```python
from build123d import *

# Parameters (mm, degrees)
SKETCH1_W           = 175
SKETCH1_H           = 2
BOSS_EXTRUDE1_DEPTH = 40
SKETCH2_W           = 2
SKETCH2_H           = 40
BOSS_EXTRUDE2_DEPTH = 50
SKETCH3_W           = 100
SKETCH3_H           = 25
BOSS_EXTRUDE3_DEPTH = 2
SKETCH4_R           = 2.5
CUT_EXTRUDE1_DEPTH  = 2
SKETCH5_W           = 12
SKETCH5_H           = 12
CUT_EXTRUDE2_DEPTH  = 2
FILLET1_R           = 5
SKETCH6_R           = 1.6
CUT_EXTRUDE3_DEPTH  = 2
BOSS_EXTRUDE4_DEPTH = 48
SHELL1_DEPTH        = 5.751288694
SHELL1_START        = 4
SHELL1_2_DEPTH      = 1.751288694
SHELL1_START_2      = 129
SHELL1_3_DEPTH      = 44
SKETCH8_R           = 5
SKETCH8_R_2         = 2.383029524
CUT_EXTRUDE4_DEPTH  = 44
SKETCH10_W          = 44
SKETCH10_H          = 28
CUT_EXTRUDE5_DEPTH  = 2
BOSS_EXTRUDE5_REACH = 146.017
SKETCH12_W          = 5.470592624
SKETCH12_H          = 9.51694338
SKETCH12_W_2        = 4.594349632
SKETCH12_H_2        = 8.868192378
CUT_EXTRUDE6_DEPTH  = 188.459328922
SKETCH13_W          = 40
SKETCH13_H          = 2
BOSS_EXTRUDE6_DEPTH = 2
SKETCH14_W          = 3
SKETCH14_H          = 2
BOSS_EXTRUDE7_DEPTH = 2
FILLET3_R           = 5
FILLET4_R           = 5


with BuildPart() as part:
    # Sketch1 → Boss-Extrude1 (new body)
    with BuildSketch(Plane.XY):
        with Locations((87.5, 1)):
            Rectangle(SKETCH1_W, SKETCH1_H)
    extrude(amount=BOSS_EXTRUDE1_DEPTH)

    # Sketch2 → Boss-Extrude2 (add)
    with BuildSketch(Plane.XZ):
        with Locations((1, 20)):
            Rectangle(SKETCH2_W, SKETCH2_H)
    extrude(amount=BOSS_EXTRUDE2_DEPTH)

    # Sketch3 → Boss-Extrude3 (add)
    with BuildSketch(Plane.XY.offset(40)):
        with Locations((52, -12.5)):
            Rectangle(SKETCH3_W, SKETCH3_H)
    extrude(amount=-BOSS_EXTRUDE3_DEPTH)

    # Sketch4 → Cut-Extrude1 (cut)
    with BuildSketch(Plane.ZY):
        with Locations((7.5, -8.5)):
            Circle(SKETCH4_R)
        with Locations((32.5, -42.5)):
            Circle(SKETCH4_R)
    extrude(amount=-CUT_EXTRUDE1_DEPTH, mode=Mode.SUBTRACT)

    # Sketch5 → Cut-Extrude2 (cut)
    with BuildSketch(Plane.XY.offset(40)):
        with Locations((21, -12.5)):
            Rectangle(SKETCH5_W, SKETCH5_H)
        with Locations((41, -12.5)):
            Rectangle(SKETCH5_W, SKETCH5_H)
        with Locations((61, -12.5)):
            Rectangle(SKETCH5_W, SKETCH5_H)
        with Locations((81, -12.5)):
            Rectangle(SKETCH5_W, SKETCH5_H)
    extrude(amount=-CUT_EXTRUDE2_DEPTH, mode=Mode.SUBTRACT)

    # Fillet1
    fillet1_edges = [part.edges().sort_by_distance(p)[0] for p in [
        (175, 1, 40),
        (1, -50, 0),
        (1, -50, 40),
        (102, -25, 39),
        (175, 1, 0),
    ]]
    fillet(fillet1_edges, radius=FILLET1_R)

    # Sketch6 → Cut-Extrude3 (cut)
    with BuildSketch(Plane(origin=(0, 2, 0), x_dir=(1, 0, 0), z_dir=(0, 1, 0))):
        with Locations(Location((17.323948769, -8, 0), (0, 0, 270))):
            Circle(SKETCH6_R)
        with Locations(Location((60.523948769, -8, 0), (0, 0, 270))):
            Circle(SKETCH6_R)
        with Locations(Location((17.323948769, -28.3, 0), (0, 0, 270))):
            Circle(SKETCH6_R)
        with Locations(Location((60.523948769, -28.3, 0), (0, 0, 270))):
            Circle(SKETCH6_R)
    extrude(amount=-CUT_EXTRUDE3_DEPTH, mode=Mode.SUBTRACT)

    # Sketch7 → Boss-Extrude4 (add)
    with BuildSketch(Plane(origin=(127, 0, 0), x_dir=(0, 0, -1), z_dir=(1, 0, 0))):
        Polygon((0, 6.905989232), (-40, 30), (-40, 2), (0, 2), align=None)
    extrude(amount=BOSS_EXTRUDE4_DEPTH)

    # Shell1: read off the stored shape, not the designer's step
    # Shell1 outline → Shell1 (cut)
    with BuildSketch(Plane(origin=(0, 0, 0), x_dir=(1, 0, 0), z_dir=(0, 1, 0))):
        with BuildLine():
            Line((129, -38), (170, -38))
            ThreePointArc((170, -38), (172.121320344, -37.121320344), (173, -35))
            Line((173, -35), (173, -5))
            ThreePointArc((173, -5), (172.121320344, -2.878679656), (170, -2))
            Line((170, -2), (129, -2))
            Line((129, -2), (129, -38))
        make_face()
    extrude(amount=SHELL1_DEPTH, mode=Mode.SUBTRACT)

    # Shell1 2 outline → Shell1 2 (cut)
    with BuildSketch(Plane(origin=(0, 0, 0), x_dir=(1, 0, 0), z_dir=(0, 1, 0)).offset(SHELL1_START)):
        with BuildLine():
            Line((170, -38), (173, -38))
            Line((173, -38), (173, -35))
            ThreePointArc((173, -35), (172.121320344, -37.121320344), (170, -38))
        make_face()
        with BuildLine():
            ThreePointArc((170, -2), (172.121320344, -2.878679656), (173, -5))
            Line((173, -5), (173, -2))
            Line((173, -2), (170, -2))
        make_face()
    extrude(amount=SHELL1_2_DEPTH, mode=Mode.SUBTRACT)

    # Shell1 3 outline → Shell1 3 (cut)
    with BuildSketch(Plane.YZ.offset(SHELL1_START_2)):
        Polygon((26.535898385, 38), (5.751288694, 38), (5.751288694, 2), align=None)
    extrude(amount=SHELL1_3_DEPTH, mode=Mode.SUBTRACT)

    # Sketch8 → Cut-Extrude4 (cut)
    with BuildSketch(Plane(origin=(0, 5.179491924, -2.990381057), x_dir=(1, 0, 0), z_dir=(0, 0.8660254037844417, -0.49999999999999495))):
        with Locations(Location((151, -26.546994616, 0), (0, 0, 270))):
            Circle(SKETCH8_R)
        with Locations(Location((168.5, -34.546994616, 0), (0, 0, 270))):
            Circle(SKETCH8_R_2)
        with Locations(Location((133.5, -34.546994616, 0), (0, 0, 270))):
            Circle(SKETCH8_R_2)
    extrude(amount=-CUT_EXTRUDE4_DEPTH, mode=Mode.SUBTRACT)

    # Sketch10 → Cut-Extrude5 (cut)
    with BuildSketch(Plane.XY.offset(40)):
        with Locations((151, 14)):
            Rectangle(SKETCH10_W, SKETCH10_H)
    extrude(amount=-CUT_EXTRUDE5_DEPTH, mode=Mode.SUBTRACT)

    # Sketch11 → Boss-Extrude5 (add, up to next)
    with BuildSketch(Plane(origin=(129, 0, 0), x_dir=(0, 0, -1), z_dir=(1, 0, 0)), mode=Mode.PRIVATE) as boss_extrude5_sk1:
        Polygon((-38, 26.535898385), (-40, 28), (-38, 28), align=None)
    boss_extrude5_tool1 = extrude(boss_extrude5_sk1.sketch, amount=BOSS_EXTRUDE5_REACH, mode=Mode.PRIVATE) - part.part
    add(boss_extrude5_tool1.solids().sort_by_distance((129, 27.511966, 38.666667))[0])

    # Sketch12 → Cut-Extrude6 (cut, through all)
    with BuildSketch(Plane(origin=(0, 4, 0), x_dir=(1, 0, 0), z_dir=(0, 1, 0))):
        with Locations((170.264703688, -39.75847169)):
            Rectangle(SKETCH12_W, SKETCH12_H)
        with Locations((170.702825184, -6.434096189)):
            Rectangle(SKETCH12_W_2, SKETCH12_H_2)
    extrude(amount=-CUT_EXTRUDE6_DEPTH, mode=Mode.SUBTRACT)

    # Sketch13 → Boss-Extrude6 (add)
    with BuildSketch(Plane(origin=(175, 0, 0), x_dir=(0, 0, -1), z_dir=(1, 0, 0))):
        with Locations((-20, 1)):
            Rectangle(SKETCH13_W, SKETCH13_H)
    extrude(amount=-BOSS_EXTRUDE6_DEPTH)

    # Sketch14 → Boss-Extrude7 (add)
    with BuildSketch(Plane(origin=(0, 0, 0), x_dir=(-1, 0, 0), z_dir=(0, 0, -1))):
        with Locations((-171.5, 1)):
            Rectangle(SKETCH14_W, SKETCH14_H)
    extrude(amount=-BOSS_EXTRUDE7_DEPTH)

    # Fillet3
    fillet3_edges = [part.edges().sort_by_distance(p)[0] for p in [
        (129, 0, 21),
        (127, 2, 20),
    ]]
    fillet(fillet3_edges, radius=FILLET3_R)

    # Fillet4
    fillet4_edges = [part.edges().sort_by_distance(p)[0] for p in [
        (151, 5.751288694, 2),
        (150.99955806, 6.905989232, 0),
    ]]
    fillet(fillet4_edges, radius=FILLET4_R)


solid = part.part
```
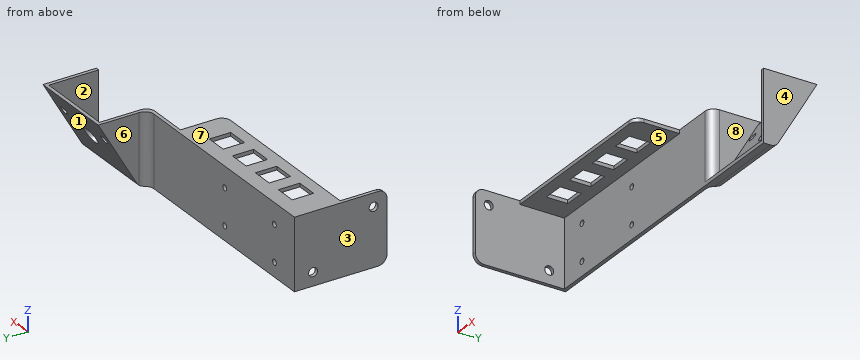
For this review, take the finished solid that the model builds, in its own axes (mm). Face numbers are marked on the shaded views. A direction names the side the tool comes from. Round coordinates to 2 decimals unless told otherwise and drop trailing zeros. Write each loop counter-clockwise with the first axis right and the second up, starting at its lowest first coordinate (ties: lowest second). Pieces come first, ordered by that corner, then holes. Notation, with made-up numbers: M 4.5,59 L 61.5,59 A17 ccw 61.5,79 Z; hole C -25.75,9 d6. An arc over 180 degrees is marked long. One line per item, written item: value. Start each with the question number.
(1) Machinability: for the marked faces 4, 5, 6, 7 and 8, which of the approach directions +Z, -Z, +X, -X, +Y, -Y give a long, thin tool a straight path to every point of the face, cutting with its end or side? Answer none if there is none.
(2) We need section C-C (x = 163.5). Give the boundary of the cut face in (y, z), and give its area (3 significant figures).
(3) We need section B-B (z = 32.5). Give the boundary of the cut face in (x, y).
(4) The part is to be moulded in two halves that separate along X. For the marked faces 1, 2 and 3, say which applies: released by +X, released by -X, zero draft, split by the parting line, or undercut.
(5) Wall thickness on line 1 (X direction, y = 13, z = 26); line 2 (Y direction, x = 17, z = 37.5); line 3 (Y direction, x = 0.95, z = 7.5): over which ranges is each line inside the solid? List them lowest first.
(6) Insertion check: pin 1 (1 mm diameter, centred on x = 129, z = 24, fed in from -Y); pin 2 (1 mm diameter, centred on x = 58.5, z = 39, fed in from +Y); pin 3 (2 mm diameter, centred on x = 29.5, z = 39.5, fed in from -Y); pin 4 (2 mm diameter, centred on y = -9, z = 7.5, fed in from -X). Each pin has a flat end and moves straight along its axis. Give the tip position at first contact, or say it passes through.
(7) We need section A-A (y = -8.5). Give the boundary of the cut face in (x, z), and give its area (3 significant figures).
(8) We need section D-D (z = 8). Give the boundary of the cut face in (x, y), and give its area (3 significant figures).
Result:
1. face 4: +Z, -Z, +X, +Y, -Y
1. face 5: -Z, +X, -Y
1. face 6: +Z, -Z, -X, +Y
1. face 7: +Z, +X, -X, +Y, -Y
1. face 8: +Z, -Y
2. outline: M 0,0 L 4.02,0 A5 ccw 8.35,2.5 L 30,40 L 28,40 L 26.54,38 L 7.19,4.5 A5 cw 2.86,2 L 0,2 Z
2. area: 102 mm²
3. outline: M 0,-50 L 2,-50 L 2,-45 L 0,-45 Z; M 0,-40 L 2,-40 L 2,0 L 124,0 A5 ccw 129,5 L 129,23.36 L 173,23.36 L 173,0 L 175,0 L 175,25.67 L 127,25.67 L 127,7 A5 cw 122,2 L 0,2 Z
4. face 1: zero draft
4. face 2: undercut
4. face 3: released by -X
5. line 1: 127 to 129, 173 to 175
5. line 2: 0 to 2
5. line 3: -50 to -11, -6 to 2
6. pin 1: y = 2.82
6. pin 2: y = 2
6. pin 3: y = -25
6. pin 4: through
7. outline: M 0,0 L 2,0 L 2,5 L 0,5 Z; M 0,10 L 2,10 L 2,38 L 15,38 L 15,40 L 0,40 Z; M 27,38 L 35,38 L 35,40 L 27,40 Z; M 47,38 L 55,38 L 55,40 L 47,40 Z; M 67,38 L 75,38 L 75,40 L 67,40 Z; M 87,38 L 102,38 L 102,40 L 87,40 Z
7. area: 174 mm²
8. outline: M 0,-50 L 2,-50 L 2,-10.95 L 0,-10.95 Z; M 0,-6.05 L 2,-6.05 L 2,0 L 15.72,0 L 15.72,2 L 0,2 Z; M 18.92,0 L 58.92,0 L 58.92,2 L 18.92,2 Z; M 62.12,0 L 124,0 A5 ccw 129,5 L 129,9.22 L 173,9.22 L 173,0 L 175,0 L 175,11.52 L 127,11.52 L 127,7 A5 cw 122,2 L 62.12,2 Z
8. area: 479 mm²
